```python
from build123d import *

# Parameters (mm, degrees)
SKETCH_1_R               = 103
SKETCH_1_R_2             = 100
EXTRUDE_1_DEPTH          = 63
SKETCH_2_R               = 103
EXTRUDE_2_DEPTH          = 2
SKETCH_4_W               = 2
SKETCH_4_H               = 60
SKETCH_4_W_2             = 120
SKETCH_4_H_2             = 2
EXTRUDE_3_DEPTH          = 10
SKETCH_5_R               = 1
SKETCH_5_W               = 70
SKETCH_5_H               = 15
CUT_EXTRUDE_1_DEPTH      = 1000
EXTRUDE_4_DEPTH          = 20
CUT_EXTRUDE_2_DEPTH      = 150
SKETCH_10_W              = 120
SKETCH_10_H              = 2
SKETCH_10_W_2            = 2
SKETCH_10_H_2            = 60
CUT_EXTRUDE_3_DEPTH      = 5
SKETCH_11_W              = 3.150152901
SKETCH_11_H              = 6.664382079
SKETCH_11_W_2            = 3.458582199
SKETCH_11_H_2            = 6.22916057
CUT_EXTRUDE_4_DEPTH      = 5
EXTRUDE_START            = 17
SKETCH_13_R              = 103
SKETCH_13_R_2            = 100
EXTRUDE_5_DEPTH          = 17
SKETCH_15_W              = 4
SKETCH_15_H              = 4.789562653
CUT_EXTRUDE_5_DEPTH      = 4
CUT_EXTRUDE_6_DEPTH      = 15
CUT_EXTRUDE_6_DEPTH_BACK = 4
SKETCH_16_W              = 4
SKETCH_16_H              = 4.789562653
EXTRUDE_START_2          = 10
SKETCH_18_R              = 103
SKETCH_18_R_2            = 100
EXTRUDE_6_DEPTH          = 10
SKETCH_19_W              = 4
SKETCH_19_H              = 4.789562653
CUT_EXTRUDE_7_DEPTH      = 10


with BuildPart() as part:
    # 草图1 → 凸台-拉伸1 (new body)
    with BuildSketch(Plane(origin=(0, 0, 0), x_dir=(1, 0, 0), z_dir=(0, 1, 0))):
        with Locations(Location((0, 0, 0), (0, 0, 270))):
            Circle(SKETCH_1_R)
        with Locations(Location((0, 0, 0), (0, 0, 270))):
            Circle(SKETCH_1_R_2, mode=Mode.SUBTRACT)
    extrude(amount=EXTRUDE_1_DEPTH)

    # 草图2 → 凸台-拉伸2 (add)
    with BuildSketch(Plane(origin=(0, 63, 0), x_dir=(1, 0, 0), z_dir=(0, 1, 0))):
        with Locations(Location((0, 0, 0), (0, 0, 270))):
            Circle(SKETCH_2_R)
    extrude(amount=EXTRUDE_2_DEPTH)

    # 草图4 → 凸台-拉伸3 (add)
    with BuildSketch(Plane.XZ.offset(-63)):
        with Locations((-66, -30)):
            Rectangle(SKETCH_4_W, SKETCH_4_H)
        with Locations((66, -30)):
            Rectangle(SKETCH_4_W, SKETCH_4_H)
        with Locations((0, 1)):
            Rectangle(SKETCH_4_W_2, SKETCH_4_H_2)
    extrude(amount=EXTRUDE_3_DEPTH)

    # 草图5 → 切除-拉伸1 (cut)
    with BuildSketch(Plane.XY.offset(2)):
        with Locations(Location((-38, 33.5, 0), (0, 0, 180))):
            Circle(SKETCH_5_R)
        with Locations(Location((38, 33.5, 0), (0, 0, 180))):
            Circle(SKETCH_5_R)
        with Locations((0, 33.5)):
            Rectangle(SKETCH_5_W, SKETCH_5_H)
    extrude(amount=CUT_EXTRUDE_1_DEPTH, mode=Mode.SUBTRACT)

    # 草图6 → 凸台-拉伸4 (add)
    with BuildSketch(Plane.XZ.offset(-63)):
        Polygon((-85, 5), (-85, 33), (53.5, 33), (53.5, 31.5), (-83.5, 31.5), (-83.5, 6.5), (53.5, 6.5), (53.5, 5), align=None)
    extrude(amount=EXTRUDE_4_DEPTH)

    # 草图7 → 切除-拉伸2 (cut)
    with BuildSketch(Plane(origin=(0, 0, 0), x_dir=(-1, 0, 0), z_dir=(0, 0, -1))):
        Polygon((-72, 63), (-67, 63), (-67, 53), (-65, 53), (-65, 63), (65, 63), (65, 53), (67, 53), (67, 63), (72, 63), (72, 23), (-72, 23), align=None)
    extrude(amount=CUT_EXTRUDE_2_DEPTH, mode=Mode.SUBTRACT)

    # 草图10 → 切除-拉伸3 (cut)
    with BuildSketch(Plane.XZ.offset(-53)):
        with Locations((0, 1)):
            Rectangle(SKETCH_10_W, SKETCH_10_H)
        with Locations((-66, -30)):
            Rectangle(SKETCH_10_W_2, SKETCH_10_H_2)
        with Locations((66, -30)):
            Rectangle(SKETCH_10_W_2, SKETCH_10_H_2)
    extrude(amount=-CUT_EXTRUDE_3_DEPTH, mode=Mode.SUBTRACT)

    # 草图11 → 切除-拉伸4 (cut)
    with BuildSketch(Plane.XZ.offset(-53)):
        with Locations((-66.11313156, -76.941337865)):
            Rectangle(SKETCH_11_W, SKETCH_11_H)
        with Locations((65.709980809, -77.158948619)):
            Rectangle(SKETCH_11_W_2, SKETCH_11_H_2)
    extrude(amount=-CUT_EXTRUDE_4_DEPTH, mode=Mode.SUBTRACT)

    # 草图13 → 凸台-拉伸5 (add)
    with BuildSketch(Plane.XZ.offset(EXTRUDE_START)):
        with Locations(Location((0, 0, 0), (0, 0, 270))):
            Circle(SKETCH_13_R)
        with Locations(Location((0, 0, 0), (0, 0, 270))):
            Circle(SKETCH_13_R_2, mode=Mode.SUBTRACT)
    extrude(amount=-EXTRUDE_5_DEPTH)

    # 草图15 → 切除-拉伸5 (cut)
    with BuildSketch(Plane.XZ.offset(17)):
        Polygon((-39, 95.331002303), (-39, 92.081485653), (-35, 92.081485653), (-35, 100), (-39, 100), align=None)
        with Locations((37, 94.476266979)):
            Rectangle(SKETCH_15_W, SKETCH_15_H)
    extrude(amount=-CUT_EXTRUDE_5_DEPTH, mode=Mode.SUBTRACT)

    # 草图16 → 切除-拉伸6 (cut, two sides: drawn at the far end of the back side and taken through both)
    with BuildSketch(Plane.XZ.offset(17).offset(-CUT_EXTRUDE_6_DEPTH_BACK)):
        with Locations((37, -94.476266979)):
            Rectangle(SKETCH_16_W, SKETCH_16_H)
        with Locations((-37, -94.476266979)):
            Rectangle(SKETCH_16_W, SKETCH_16_H)
    extrude(amount=CUT_EXTRUDE_6_DEPTH + CUT_EXTRUDE_6_DEPTH_BACK, mode=Mode.SUBTRACT)

    # 草图18 → 凸台-拉伸6 (add)
    with BuildSketch(Plane.XZ.offset(17).offset(EXTRUDE_START_2)):
        with Locations(Location((0, 0, 0), (0, 0, 270))):
            Circle(SKETCH_18_R)
        with Locations(Location((0, 0, 0), (0, 0, 270))):
            Circle(SKETCH_18_R_2, mode=Mode.SUBTRACT)
    extrude(amount=-EXTRUDE_6_DEPTH)

    # 草图19 → 切除-拉伸7 (cut)
    with BuildSketch(Plane.XZ.offset(27)):
        with Locations((-37, -94.476266979)):
            Rectangle(SKETCH_19_W, SKETCH_19_H)
        with Locations((37, -94.476266979)):
            Rectangle(SKETCH_19_W, SKETCH_19_H)
        with Locations((-37, 94.476266979)):
            Rectangle(SKETCH_19_W, SKETCH_19_H)
        with Locations((37, 94.476266979)):
            Rectangle(SKETCH_19_W, SKETCH_19_H)
    extrude(amount=-CUT_EXTRUDE_7_DEPTH, mode=Mode.SUBTRACT)


solid = part.part
```
The model under review builds one solid part; all positions refer to its coordinate system, in mm. A direction names the side the tool comes from. Round coordinates to 2 decimals unless told otherwise and drop trailing zeros. Order: outer loops, then holes, each group sorted by start corner. A loop starts at its lowest first (then second) coordinate and runs counter-clockwise, first axis right, second up.
(1) Take a section at D-D, the plane z = -88. State the section outline as (x, y) points.
Working result:
outline: (-53.53, -27) - (-47.5, -27) - (-47.5, 23) - (-53.53, 23) - close; (-53.53, 63) - (53.53, 63) - (53.53, 65) - (-53.53, 65) - close; (47.5, -27) - (53.53, -27) - (53.53, 23) - (47.5, 23) - close
(2) Take a section at C-C, the plane y = -20. State the section outline as (x, z) points.
Working result:
outline: (-39, -95.33) - (-39, -92.08) arc R100 cw to (-39, 92.08) - (-39, 95.33) arc R103 ccw to start; (-35, -96.87) arc R103 ccw to (35, -96.87) - (35, -93.67) arc R100 cw to (-35, -93.67) - close; (-35, 93.67) arc R100 cw to (35, 93.67) - (35, 96.87) arc R103 ccw to (-35, 96.87) - close; (39, -95.33) arc R103 ccw to (39, 95.33) - (39, 92.08) arc R100 cw to (39, -92.08) - close
(3) Mouldability with a two-part tool opening along Y and no side actions: class faces 4 (the face through (102, -27, 0)), 5 (the face through (-1, 61, 2)), 6 (the face through (0, 23, -101)) as released by +Y, released by -Y, zero draft, split by the parting line, or undercut.
Working result:
face 4: released by -Y
face 5: zero draft
face 6: undercut
(4) Take a section at A-A, the plane y = 55.5. State the section outline as (x, z) points, plus the area to 3 significant figures.
Working result:
outline: (-85, 5) - (53.5, 5) - (53.5, 6.5) - (-83.5, 6.5) - (-83.5, 31.5) - (53.5, 31.5) - (53.5, 33) - (-85, 33) - close; (-72, -73.65) - (-72, -69.4) arc R100 cw (long way) to (72, -69.4) - (72, -73.65) arc R103 ccw (long way) to start
area: 1,890 mm2
(5) Wall thickness on L1, parallel to Z at x = 0, y = -5.5; L2, parallel to Y at x = -38, z = 95: over which ranges is each line inside the solid? List them lowest first.
Working result:
L1: z = -103 to -100, 100 to 103
L2: y = -13 to 32.5, 34.5 to 65
(6) Take a section at B-B, the plane x = 25.5. State the section outline as (y, z) points, plus the area to 3 significant figures.
Working result:
outline: (-27, -99.79) - (23, -99.79) - (23, -96.69) - (-27, -96.69) - close; (-27, 96.69) - (26, 96.69) - (26, 99.79) - (-27, 99.79) - close; (41, 96.69) - (63, 96.69) - (63, 33) - (43, 33) - (43, 31.5) - (63, 31.5) - (63, 6.5) - (43, 6.5) - (43, 5) - (63, 5) - (63, 2) - (58, 2) - (58, 0) - (63, 0) - (63, -99.79) - (65, -99.79) - (65, 99.79) - (41, 99.79) - close
area: 857 mm2
(7) For P1, Ø4, axis at x = 4.5, y = 6, coming from the +Z side; P2, Ø3.5, axis at y = -20, z = -94.5, coming from the -X side; P3, Ø1, axis at y = -1.5, z = -40, coming from the +X side; P4, Ø1.2, axis at x = 38, y = 33.5, coming from the -Z side, all flat-tipped, find the tip position at first contact; note any pin that passes through.
Working result:
P1: stops at z = 102.97
P2: stops at x = -44.79
P3: stops at x = 95.12
P4: passes through
(8) Tool access review of faces 1 (the face through (0, 26, 101)), 2 (the face through (-14, 53, 31.5)), 3 (the face through (-65, 61, -30)): name each direction out of +Z, -Z, +X, -X, +Y, -Y from which nothing blocks a thin tool from reaching the whole face with its end or side.
Working result:
face 1: +Z, -Z
face 2: -Y
face 3: -Z, -Y
